Here's how the part is built. I have some questions about the finished solid (model axes, mm). A direction names the side the tool comes from. Round coordinates to 2 decimals unless told otherwise and drop trailing zeros. Loops run counter-clockwise (first coordinate to the right, second up) from the corner with the lowest first, then second, coordinate; pieces in that order, holes last. Notation, with made-up numbers: M 65.25,47.5 L 106.25,47.5 A25 ccw 106.25,64.5 Z; hole C -22,10.5 d2. An arc over 180 degrees is marked long. Put each result on its own line as item: value. Start each with the question number.
```python
from build123d import *

# Parameters (mm, degrees)
F1_DEPTH = 30


with BuildPart() as f1:
    # F0 (on Front) → F1 (new body)
    with BuildSketch(Plane.XZ):
        with BuildLine():
            Line((-100, 30.548105), (-100, -39.451895))
            Line((-100, -39.451895), (-70, -39.451895))
            Line((-70, -39.451895), (-70, -19.451895))
            ThreePointArc((-70, -19.451895), (-67.071068, -12.380827), (-60, -9.451895))
            ThreePointArc((-60, -9.451895), (-52.928932, -12.380827), (-50, -19.451895))
            Line((-50, -19.451895), (-50, -39.451895))
            Line((-50, -39.451895), (10, -39.451895))
            Line((10, -39.451895), (10, -19.451895))
            ThreePointArc((10, -19.451895), (12.928932, -12.380827), (20, -9.451895))
            ThreePointArc((20, -9.451895), (27.071068, -12.380827), (30, -19.451895))
            Line((30, -19.451895), (30, -39.451895))
            Line((30, -39.451895), (70, -39.451895))
            Line((70, -39.451895), (70, 4.548105))
            Line((70, 4.548105), (35, 50.548105))
            Line((35, 50.548105), (0, 50.548105))
            Line((0, 50.548105), (0, 20.548105))
            ThreePointArc((0, 20.548105), (-15, 5.548105), (-30, 20.548105))
            Line((-30, 20.548105), (-30, 50.548105))
            Line((-30, 50.548105), (-80, 50.548105))
            ThreePointArc((-80, 50.548105), (-94.142136, 44.69024), (-100, 30.548105))
        make_face()
    extrude(amount=F1_DEPTH)


solid = f1.part
```
1) On a 3-axis mill with a long thin cutter (end or side, diameter ignored), from which of +Z, -Z, +X, -X, +Y, -Y can I reach the whole of each face in a straight line? I mean faces 4 (the face through (-70, -15, -30)), 5 (the face through (18, -15, 50.548)), 6 (the face through (0, -15, 36)). Say none if no direction works.
2) Suppose I cut it at D-D (z = 44.5). Write out the boundary of the cut face in (x, y).
3) Suppose I cut it at C-C (x = -15). Write out the boundary of the cut face in (y, z), plus the area to 3 significant figures.
4) Suppose I cut it at B-B (z = 17). Write out the boundary of the cut face in (x, y), plus the area to 3 significant figures.
5) Suppose I cut it at A-A (y = -25.5). Write out the boundary of the cut face in (x, z).
6) If we mould it in two halves opening along X, with no side actions, what happens to faces 1 (the face through (-55, -15, 50.548)), 2 (the face through (70, -15, -18)), 3 (the face through (30, -15, -29))? For each: pulls with the +X half, pulls with the -X half, needs draft (parallel to the pull), parting line crosses it, or undercut.
7) I'm going to push flat-ended pins straight in: P1, Ø1, axis at x = -65, z = 35, coming from the +Y side; P2, Ø5, axis at y = -22, z = 40.5, coming from the +X side; P3, Ø1.5, axis at x = -12.5, y = -9.5, coming from the +Z side. Where does each tip first touch, or does it pass through?
8) If I drill on probe 1 along X at (y, z) = (-23.5, -34); probe 2 along X at (y, z) = (-7.25, -13); probe 3 along X at (y, z) = (-8.5, 8), over which ranges is the centre line in solid material (lowest first)? Write a range as from..to.
Results are:
1. face 4: -Z, +Y, -Y
1. face 5: +Z, +X, -X, +Y, -Y
1. face 6: +Z, +Y, -Y
2. outline: M -94.33,-30 L -30,-30 L -30,0 L -94.33,0 Z; M 0,-30 L 39.6,-30 L 39.6,0 L 0,0 Z
3. outline: M -30,-39.45 L 0,-39.45 L 0,5.55 L -30,5.55 Z
3. area: 1,350 mm²
4. outline: M -100,-30 L -29.57,-30 L -29.57,0 L -100,0 Z; M -0.43,-30 L 60.53,-30 L 60.53,0 L -0.43,0 Z
4. area: 3,940 mm²
5. outline: M -100,-39.45 L -70,-39.45 L -70,-19.45 A10 cw -60,-9.45 A10 cw -50,-19.45 L -50,-39.45 L 10,-39.45 L 10,-19.45 A10 cw 20,-9.45 A10 cw 30,-19.45 L 30,-39.45 L 70,-39.45 L 70,4.55 L 35,50.55 L 0,50.55 L 0,20.55 A15 cw -30,20.55 L -30,50.55 L -80,50.55 A20 ccw -100,30.55 Z
6. face 1: needs draft
6. face 2: pulls with the +X half
6. face 3: undercut
7. P1: y = 0
7. P2: x = 44.55
7. P3: z = 5.9
8. probe 1: -100..-70, -50..10, 30..70
8. probe 2: -100..-67.64, -52.36..12.36, 27.64..70
8. probe 3: -100..-23.22, -6.78..67.37
